For this review, take the finished solid that the model builds, in its own axes (mm). Face numbers are marked on the shaded views. Give positions to 0.01 mm unless a question says otherwise; leave off trailing zeros. Order: outer loops, then holes, each group sorted by start corner. A loop starts at its lowest first (then second) coordinate and runs counter-clockwise, first axis right, second up. Notation, with made-up numbers: (37, 61.25) - (67, 61.25) arc R10 cw to (67, 76.25) - close; hole circle Ø11 at (85.25, -37). An arc over 180 degrees is marked (long way). Put each result on its own line as item: value. Start each with the question number.
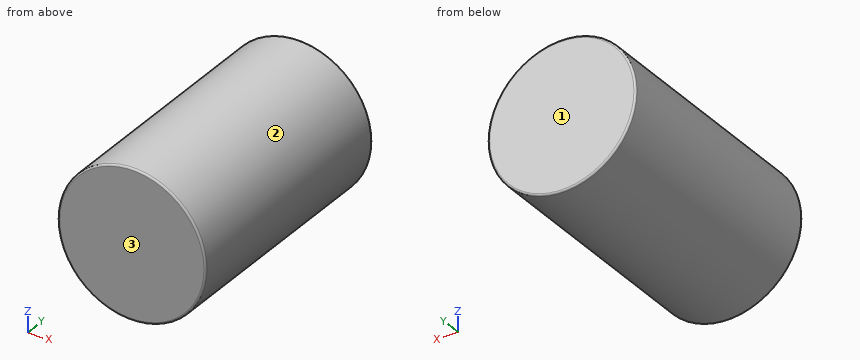
```python
from build123d import *

# Parameters (mm, degrees)
SKETCH_1_R      = 4
EXTRUDE_1_DEPTH = 13.5
FILLET_1_R      = 0.1
FILLET_2_R      = 0.1


with BuildPart() as part:
    # Эскиз1 → Бобышка-Вытянуть1 (new body)
    with BuildSketch(Plane(origin=(0, 0, 0), x_dir=(1, 0, 0), z_dir=(0, 1, 0))):
        Circle(SKETCH_1_R)
    extrude(amount=EXTRUDE_1_DEPTH)

    # Скругление1
    fillet_1_edges = [part.edges().sort_by_distance(p)[0] for p in [
        (-4, 13.5, 0),
    ]]
    fillet(fillet_1_edges, radius=FILLET_1_R)

    # Скругление2
    fillet_2_edges = [part.edges().sort_by_distance(p)[0] for p in [
        (-4, 0, 0),
    ]]
    fillet(fillet_2_edges, radius=FILLET_2_R)


solid = part.part
```
1. Wall thickness on line 1 (Z direction, x = -3.25, y = 10); line 2 (X direction, y = 0.75, z = -2.5); line 3 (X direction, y = 3.5, z = 1.75): over which ranges is each line inside the solid? List them lowest first. Write a range as from..to.
2. Add section A-A, the plane y = 5.75. Give the boundary of the cut face in (x, z).
3. Clearance check with flat-ended pins moving along their axes: pin 1 (1 mm diameter, centred on y = 5, z = -2, fed in from -X); pin 2 (2 mm diameter, centred on x = 1.5, y = 2.5, fed in from +Z). State where each tip first meets the part, or that it passes through.
4. The part is to be moulded in two halves that separate along Y. For the marked faces 1, 2 and 3, say which applies: released by +Y, released by -Y, zero draft, split by the parting line, or undercut.
Found:
1. line 1: z = -2.33..2.33
1. line 2: x = -3.12..3.12
1. line 3: x = -3.6..3.6
2. outline: circle Ø8 at (0, 0)
3. pin 1: stops at x = -3.71
3. pin 2: stops at z = 3.97
4. face 1: released by +Y
4. face 2: zero draft
4. face 3: released by -Y
